```python
from build123d import *

# Parameters (mm, degrees)
F0_W     = 100
F0_H     = 200
F1_DEPTH = 10
F2_W     = 50
F2_H     = 40
F3_DEPTH = 25
F4_R     = 12.5
F5_DEPTH = 10.001


with BuildPart() as f1:
    # F0 (on Top) → F1 (new body)
    with BuildSketch(Plane.XY):
        with Locations((-17.348269, 5.148082)):
            Rectangle(F0_W, F0_H)
    extrude(amount=F1_DEPTH)

    # F2 (on Top) → F3 (join)
    with BuildSketch(Plane.XY):
        with Locations((-42.348269, 85.148082)):
            Rectangle(F2_W, F2_H)
    extrude(amount=F3_DEPTH)

    # F4 (on face) → F5 (cut, through all)
    with BuildSketch(Plane.XY.offset(10)):
        with Locations((-2.348269, -64.851918)):
            Circle(F4_R)
    extrude(amount=-F5_DEPTH, mode=Mode.SUBTRACT)


solid = f1.part
```
The model under review builds one solid part; all positions refer to its coordinate system, in mm. A direction names the side the tool comes from. Give positions to 0.01 mm unless a question says otherwise; leave off trailing zeros. Write each loop counter-clockwise with the first axis right and the second up, starting at its lowest first coordinate (ties: lowest second). Pieces come first, ordered by that corner, then holes. Notation, with made-up numbers: (-21, 10.5) - (30, 10.5) arc R23 cw to (30, 23.5) - close; hole circle Ø5 at (-6, -24.5). An arc over 180 degrees is marked (long way). Answer in a Markdown table with one row per item. Add a question column.
1. We need section D-D on z = 2.25. Write out the cut boundary in (x, y).
2. We need section B-B on x = -13. Write out the cut boundary in (y, z).
3. Insertion check: P1, Ø4, axis at x = -34, z = 19, coming from the -Y side; P2, Ø10, axis at x = -23.5, y = 21, coming from the +Z side; P3, Ø12, axis at y = 87, z = 17.5, coming from the +X side. Each pin has a flat end and moves straight along its axis. Give the tip position at first contact, or say it passes through.
4. Tool access review of faces 1 (the cylindrical face through (-3.98, -52.46, 5.07)), 2 (the flat face through (-17.348, 85, 17)), 3 (the flat face through (-43, 65.148, 17)): name each direction out of +Z, -Z, +X, -X, +Y, -Y from which nothing blocks a thin tool from reaching the whole face with its end or side.
5. We need section A-A on y = -70.5. Write out the cut boundary in (x, z).
6. We need section C-C on x = -29. Write out the cut boundary in (y, z).
7. Wall thickness on line 1 along X through (y, z) = (-65.5, 9); line 2 along Z through (x, y) = (15.5, -77.5); line 3 along Y through (x, z) = (-46.5, 16): over which ranges is each line inside the solid? List them lowest first. Write a range as [from, to].
Ans:
| question | item | result |
|---|---|---|
| 1 | outline | (-67.35, -94.85) - (32.65, -94.85) - (32.65, 105.15) - (-67.35, 105.15) - close; hole circle Ø25 at (-2.35, -64.85) |
| 2 | outline | (-94.85, 0) - (-71.39, 0) - (-71.39, 10) - (-94.85, 10) - close; (-58.31, 0) - (105.15, 0) - (105.15, 10) - (-58.31, 10) - close |
| 3 | P1 | stops at y = 65.15 |
| 3 | P2 | stops at z = 10 |
| 3 | P3 | stops at x = -17.35 |
| 4 | face 1 | +Z, -Z |
| 4 | face 2 | +Z, +X, +Y, -Y |
| 4 | face 3 | +Z, +X, -X, -Y |
| 5 | outline | (-67.35, 0) - (-13.5, 0) - (-13.5, 10) - (-67.35, 10) - close; (8.8, 0) - (32.65, 0) - (32.65, 10) - (8.8, 10) - close |
| 6 | outline | (-94.85, 0) - (105.15, 0) - (105.15, 25) - (65.15, 25) - (65.15, 10) - (-94.85, 10) - close |
| 7 | line 1 | x = [-67.35, -14.83], [10.13, 32.65] |
| 7 | line 2 | z = [0, 10] |
| 7 | line 3 | y = [65.15, 105.15] |
